Can you work these out from the model? Positions are in its coordinate system, mm. A direction names the side the tool comes from. Give positions to 0.01 mm unless a question says otherwise; leave off trailing zeros. Loops run counter-clockwise (first coordinate to the right, second up) from the corner with the lowest first, then second, coordinate; pieces in that order, holes last. Notation, with made-up numbers: (-2.75, 26.5) -> (43.25, 26.5) arc R29 cw to (43.25, 55.5) -> close; hole circle Ø1 at (-21, 56). An arc over 180 degrees is marked (long way). Return JSON: item names as keys, results as strings. Group by question number.
Q1. Suppose I cut it at C-C, the plane y = 0.5. Please give me the cut outline in (x, z), and give its area (3 significant figures).
Q2. Which directions (+Z, -Z, +X, -X, +Y, -Y) give clear straight access to the entire face, cutting with the end or side of a thin tool? Please do faces 1 (the cylindrical face through (2.737, 6.041, -9.618)), 2 (the flat face through (-13.61, 2.46, 5.64)).
Q3. Suppose I cut it at B-B, the plane z = 0. Please give me the cut outline in (x, y), and give its area (3 significant figures).
Q4. Will these pins go through, and if not, where does the flat tip stop? pin 1 (2 mm diameter, centred on x = -11.5, z = 3.5, fed in from +Y); pin 2 (1 mm diameter, centred on x = 8, y = 4.5, fed in from -Z); pin 3 (4 mm diameter, centred on x = -10, y = 7.5, fed in from -Z).
Q5. Thinking about a two-plate mould opening in Z: for faces 3 (the flat face through (-13.6, 5, 1.7)), 4 (the flat face through (-13.388, 2.465, -5.713)), 5 (the cylindrical face through (18.727, 2.465, -0.358)), 6 (the flat face through (13.388, 2.465, 5.713)), which applies, pulls with the +Z half, pulls with the -Z half, needs draft (parallel to the pull), parting line crosses it, or undercut?
Q6. Suppose I cut it at A-A, the plane x = 0. Please give me the cut outline in (y, z).
Q7. I need wall thicknesses on line 1 along X through (y, z) = (3.85, 0); line 2 along Y through (x, z) = (-20, -1); line 3 along Z through (x, y) = (-18.5, 2.75). Which ranges of each line are inside material? Lowest first, please. Write a range as [from, to].
Q8. Suppose I cut it at D-D, the plane x = 14. Please give me the cut outline in (y, z).
```python
from build123d import *

# Parameters (mm, degrees)
SKETCH1_R             = 2.75
BOSS_EXTRUDE1_DEPTH   = 5
BOSS_EXTRUDE1_2_DEPTH = 5
SKETCH1_3_R           = 10
BOSS_EXTRUDE2_DEPTH   = 10
SKETCH2_R             = 4
CUT_EXTRUDE1_DEPTH    = 26.734218465


with BuildPart() as part:
    # Sketch1 → Boss-Extrude1 (new body)
    with BuildSketch(Plane(origin=(0, 0, 0), x_dir=(1, 0, 0), z_dir=(0, 1, 0))):
        with BuildLine():
            Line((21.5, -3), (21.5, 3))
            Line((21.5, 3), (5.5, 8.351646544))
            ThreePointArc((5.5, 8.351646544), (8.803408431, 4.74341649), (10, 0))
            ThreePointArc((10, 0), (8.803408431, -4.74341649), (5.5, -8.351646544))
            Line((5.5, -8.351646544), (21.5, -3))
        make_face()
        with Locations(Location((16, 0, 0), (0, 0, 270))):
            Circle(SKETCH1_R, mode=Mode.SUBTRACT)
    extrude(amount=BOSS_EXTRUDE1_DEPTH)



with BuildPart() as body_2:
    # Sketch1 → Boss-Extrude1 2 (new body)
    with BuildSketch(Plane(origin=(0, 0, 0), x_dir=(1, 0, 0), z_dir=(0, 1, 0))):
        with BuildLine():
            ThreePointArc((-5.5, -8.351646544), (-10, 0), (-5.5, 8.351646544))
            Line((-5.5, 8.351646544), (-21.5, 3))
            Line((-21.5, 3), (-21.5, -3))
            Line((-21.5, -3), (-5.5, -8.351646544))
        make_face()
        with Locations(Location((-16, 0, 0), (0, 0, 270))):
            Circle(SKETCH1_R, mode=Mode.SUBTRACT)
    extrude(amount=BOSS_EXTRUDE1_2_DEPTH)


with BuildPart() as part_1:
    add(part.part)

    add(body_2.part)  # Boss-Extrude2 merges body 2
    # Sketch1_3 → Boss-Extrude2 (add)
    with BuildSketch(Plane(origin=(0, 0, 0), x_dir=(1, 0, 0), z_dir=(0, 1, 0))):
        with Locations(Location((0, 0, 0), (0, 0, 56.632987031))):
            Circle(SKETCH1_3_R)
    extrude(amount=BOSS_EXTRUDE2_DEPTH)

    # Sketch2 → Cut-Extrude1 (cut, through all)
    with BuildSketch(Plane(origin=(0, 10, 0), x_dir=(1, 0, 0), z_dir=(0, 1, 0))):
        with Locations(Location((0, 0, 0), (0, 0, 270))):
            Circle(SKETCH2_R)
    extrude(amount=-CUT_EXTRUDE1_DEPTH, mode=Mode.SUBTRACT)


solid = part_1.part
```
Ans:
{
 "1": {"outline": "(-21.5, -3) -> (-5.5, -8.35) arc R10 ccw to (5.5, -8.35) -> (21.5, -3) -> (21.5, 3) -> (5.5, 8.35) arc R10 ccw to (-5.5, 8.35) -> (-21.5, 3) -> close; hole circle Ø5.5 at (-16, 0); hole circle Ø8 at (0, 0); hole circle Ø5.5 at (16, 0)", "area": "474 mm^2"},
 "2": {"face 1": "+Y", "face 2": "+Z, -X, +Y, -Y"},
 "3": {"outline": "(-21.5, 0) -> (-18.75, 0) -> (-18.75, 5) -> (-21.5, 5) -> close; (-13.25, 0) -> (-4, 0) -> (-4, 10) -> (-10, 10) -> (-10, 5) -> (-13.25, 5) -> close; (4, 0) -> (13.25, 0) -> (13.25, 5) -> (10, 5) -> (10, 10) -> (4, 10) -> close; (18.75, 0) -> (21.5, 0) -> (21.5, 5) -> (18.75, 5) -> close", "area": "180 mm^2"},
 "4": {"pin 1": "stops at y = 5", "pin 2": "stops at z = -7.68", "pin 3": "stops at z = -6"},
 "5": {"face 3": "needs draft", "face 4": "pulls with the -Z half", "face 5": "undercut", "face 6": "pulls with the +Z half"},
 "6": {"outline": "(0, -10) -> (10, -10) -> (10, -4) -> (0, -4) -> close; (0, 4) -> (10, 4) -> (10, 10) -> (0, 10) -> close"},
 "7": {"line 1": "x = [-21.5, -18.75], [-13.25, -4], [4, 13.25], [18.75, 21.5]", "line 2": "y = [0, 5]", "line 3": "z = [-4, -1.15], [1.15, 4]"},
 "8": {"outline": "(0, -5.51) -> (5, -5.51) -> (5, -1.89) -> (0, -1.89) -> close; (0, 1.89) -> (5, 1.89) -> (5, 5.51) -> (0, 5.51) -> close"}
}
